from build123d import *

# Parameters (mm, degrees)
SKETCH1_W           = 40
SKETCH1_H           = 30
BOSS_EXTRUDE1_DEPTH = 10
SKETCH2_R           = 4.05
CUT_EXTRUDE1_DEPTH  = 10
SKETCH3_W           = 15
SKETCH3_H           = 15
SKETCH3_R           = 4.05
BOSS_EXTRUDE2_DEPTH = 30
SKETCH4_R           = 1.45
CUT_EXTRUDE2_DEPTH  = 5
CHAMFER1_SIZE       = 5
SKETCH5_R           = 16.957046222
CUT_EXTRUDE3_DEPTH  = 10


with BuildPart() as part:
    # Sketch1 → Boss-Extrude1 (new body)
    with BuildSketch(Plane(origin=(0, 0, 0), x_dir=(1, 0, 0), z_dir=(0, 1, 0))):
        Polygon((14.142135624, -40), (0, -40), (7.071067812, -47.071067812), (0, -54.142135624), (35.355339059, -89.497474683), (49.497474683, -75.355339059), align=None)
        Polygon((7.071067812, -47.071067812), (0, -40), (-7.071067812, -47.071067812), (0, -54.142135624), align=None)
        Polygon((0, -40), (-14.142135624, -40), (-49.497474683, -75.355339059), (-35.355339059, -89.497474683), (0, -54.142135624), (-7.071067812, -47.071067812), align=None)
        Polygon((10, 40), (-10, 40), (-40, 25), (-40, 15), (-40, -15), (-14.142135624, -40), (-7.071067812, -32.928932188), (0, -40), (7.071067812, -32.928932188), (14.142135624, -40), (40, -15), (40, 15), (40, 25), align=None)
        Polygon((7.071067812, -32.928932188), (0, -40), (14.142135624, -40), align=None)
        Polygon((-7.071067812, -32.928932188), (-14.142135624, -40), (0, -40), align=None)
        with Locations((-60, 0)):
            Rectangle(SKETCH1_W, SKETCH1_H)
        with Locations((60, 0)):
            Rectangle(SKETCH1_W, SKETCH1_H)
    extrude(amount=BOSS_EXTRUDE1_DEPTH)

    # Sketch2 → Cut-Extrude1 (cut)
    with BuildSketch(Plane(origin=(0, 10, 0), x_dir=(1, 0, 0), z_dir=(0, 1, 0))):
        with Locations((0, 20)):
            Circle(SKETCH2_R)
    extrude(amount=-CUT_EXTRUDE1_DEPTH, mode=Mode.SUBTRACT)

    # Sketch3 → Boss-Extrude2 (add)
    with BuildSketch(Plane(origin=(0, 10, 0), x_dir=(1, 0, 0), z_dir=(0, 1, 0))):
        with Locations((0, 20)):
            Rectangle(SKETCH3_W, SKETCH3_H)
        with Locations((0, 20)):
            Circle(SKETCH3_R, mode=Mode.SUBTRACT)
    extrude(amount=BOSS_EXTRUDE2_DEPTH)

    # Sketch4 → Cut-Extrude2 (cut)
    with BuildSketch(Plane(origin=(0, 0, -27.5), x_dir=(-1, 0, 0), z_dir=(0, 0, -1))):
        with Locations((0, 35)):
            Circle(SKETCH4_R)
        with Locations((0, 20)):
            Circle(SKETCH4_R)
    extrude(amount=-CUT_EXTRUDE2_DEPTH, mode=Mode.SUBTRACT)

    # Chamfer1
    chamfer1_edges = [part.edges().sort_by_distance(p)[0] for p in [
        (7.5, 10, -20),
        (7.5, 25, -12.5),
        (-7.5, 10, -20),
        (0, 10, -12.5),
        (-7.5, 25, -12.5),
    ]]
    chamfer(chamfer1_edges, length=CHAMFER1_SIZE)

    # Sketch5 → Cut-Extrude3 (cut)
    with BuildSketch(Plane(origin=(0, 10, 0), x_dir=(1, 0, 0), z_dir=(0, 1, 0))):
        with Locations((0, -13.19116881)):
            Circle(SKETCH5_R)
    extrude(amount=-CUT_EXTRUDE3_DEPTH, mode=Mode.SUBTRACT)


solid = part.part
Verification items for the finished model (mm, model axes). A direction names the side the tool comes from. Give positions to 0.01 mm unless a question says otherwise; leave off trailing zeros. Write each loop counter-clockwise with the first axis right and the second up, starting at its lowest first coordinate (ties: lowest second). Pieces come first, ordered by that corner, then holes.
(1) Cross-section at B-B (z = 80.5). Enter the section's corners in (x, y), plus the area to 3 significant figures.
(2) Gauge pin test, flat ends, axial feed: pin 1 (3 mm diameter, centred on x = -68, y = 6.5, fed in from -Z); pin 2 (4 mm diameter, centred on x = 0, y = 26.5, fed in from +Z); pin 3 (3 mm diameter, centred on y = 25.5, z = -23, fed in from +X); pin 4 (5 mm diameter, centred on x = 0, z = -20, fed in from +Y) (3 decimals). Record the tip position at first contact, or that the pin passes through.
(3) Material ranges on line 1 (X direction, y = 20, z = -24); line 2 (Z direction, x = 0, y = 22); line 3 (Y direction, x = 0, z = -26.2), recorded low to high.
(4) Access from +Z, -Z, +X, -X, +Y, -Y to the whole of each face (thin tool, end or side, straight path). Record for faces 4 (the face through (-7.5, 27, -22)), 5 (the face through (-40, 5, -20)), 6 (the face through (17.43, 4.93, 71.57)).
(5) Mould release check, pull along X, two halves, no side actions. Record for faces 1 (the face through (0, 27, -12.5)), 2 (the face through (7.5, 27, -22)), 3 (the face through (-0.878, 19.72, -16.046)): +X half, -X half, draft (parallel to the pull), parting line (faces both ways), or undercut.
(6) Cross-section at A-A (z = -20). Enter the section's corners in (x, y), plus the area to 3 significant figures.
Worked out:
1. outline: (-44.35, 0) - (-26.36, 0) - (-26.36, 10) - (-44.35, 10) - close; (26.36, 0) - (44.35, 0) - (44.35, 10) - (26.36, 10) - close
1. area: 360 mm2
2. pin 1: stops at z = -15
2. pin 2: stops at z = -12.5
2. pin 3: stops at x = 7.5
2. pin 4: passes through
3. line 1: x = -7.5 to -1.45, 1.45 to 7.5
3. line 2: z = -27.5 to -24.05, -15.95 to -12.5
3. line 3: y = 0 to 18.55, 21.45 to 33.55, 36.45 to 40
4. face 4: +Z, -Z, -X, +Y
4. face 5: -Z, -X, +Y, -Y
4. face 6: +Z, +Y, -Y
5. face 1: draft
5. face 2: +X half
5. face 3: undercut
6. outline: (-40, 0) - (-4.05, 0) - (-4.05, 40) - (-7.5, 40) - (-7.5, 15) - (-12.5, 10) - (-40, 10) - close; (4.05, 0) - (40, 0) - (40, 10) - (12.5, 10) - (7.5, 15) - (7.5, 40) - (4.05, 40) - close
6. area: 951 mm2
